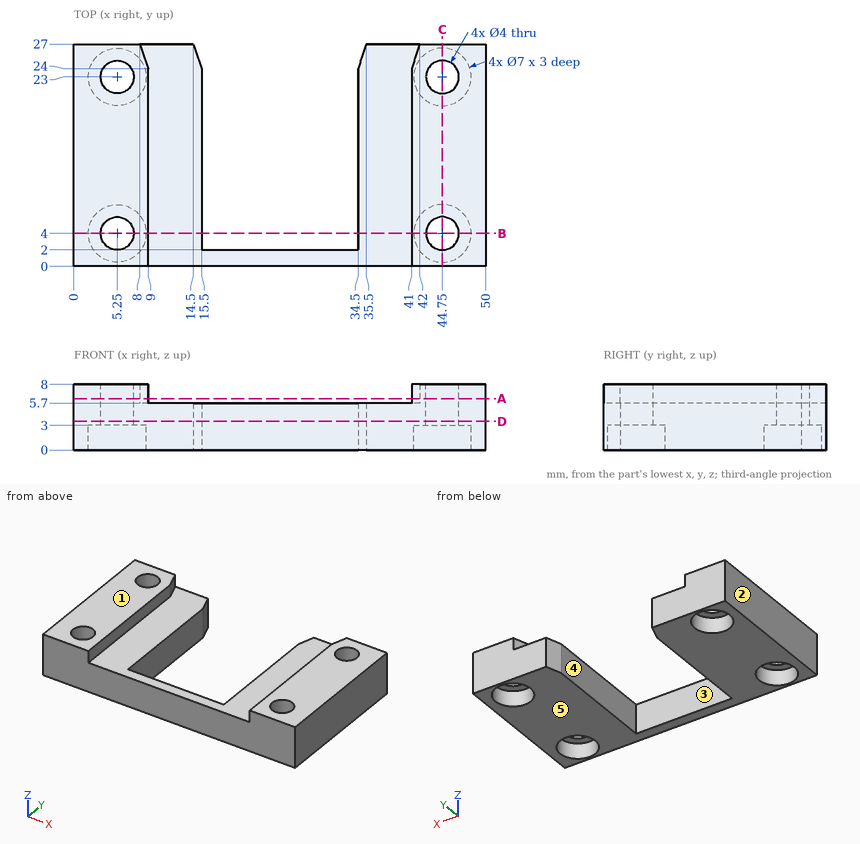
Job drawing, mm, ordinate dimensions from the low corner. One solid piece. A direction names the side the tool comes from. Round coordinates to 2 decimals unless told otherwise and drop trailing zeros. Loops run counter-clockwise (first coordinate to the right, second up) from the corner with the lowest first, then second, coordinate; pieces in that order, holes last.
(1) Cut at B-B (y = 4). Give the cut face in (x, z), plus the area to 3 significant figures.
(2) Cut at D-D (z = 3.5). Give the cut face in (x, y), plus the area to 3 significant figures.
(3) Drop flat-ended pins along their axis: pin 1 (4.5 mm diameter, centred on x = 26, z = 3.5, fed in from +Y); pin 2 (1.5 mm diameter, centred on x = 32, y = 20, fed in from -Z); pin 3 (3.5 mm diameter, centred on x = 6.5, y = 5, fed in from -Z). Give the stop position or say it passes through.
(4) Cut at A-A (z = 6.25). Give the cut face in (x, y).
(5) Two-plate mould, pull along X, no slides. Class the marked faces 1, 2 and 3: +X half, -X half, draft (parallel to the pull), parting line (faces both ways), or undercut.
(6) Wall check: line 1 along Y through (x, z) = (44.75, 2.2); line 2 along X through (y, z) = (4, 6.3); line 3 along Y through (x, z) = (44.75, 5.85). Give the ranges that are in metal, low to high.
(7) Cut at C-C (x = 44.75). Give the cut face in (y, z).
(8) Which spindle directions (+Z, -Z, +X, -X, +Y, -Y) get a long thin tool onto all of the face, cutting with end or side? Do the marked faces 4 and 5. Say none if no direction does.
Findings below:
1. outline: (0, 0) - (1.75, 0) - (1.75, 3) - (3.25, 3) - (3.25, 8) - (0, 8) - close; (7.25, 3) - (8.75, 3) - (8.75, 0) - (15.5, 0) - (15.5, 5.7) - (9, 5.7) - (9, 8) - (7.25, 8) - close; (34.5, 0) - (41.25, 0) - (41.25, 3) - (42.75, 3) - (42.75, 8) - (41, 8) - (41, 5.7) - (34.5, 5.7) - close; (46.75, 3) - (48.25, 3) - (48.25, 0) - (50, 0) - (50, 8) - (46.75, 8) - close
1. area: 136 mm2
2. outline: (0, 0) - (50, 0) - (50, 27) - (35.5, 27) - (34.5, 24) - (34.5, 2) - (15.5, 2) - (15.5, 24) - (14.5, 27) - (0, 27) - close; hole circle Ø4 at (5.25, 4); hole circle Ø4 at (5.25, 23); hole circle Ø4 at (44.75, 4); hole circle Ø4 at (44.75, 23)
2. area: 822 mm2
3. pin 1: stops at y = 2
3. pin 2: passes through
3. pin 3: stops at z = 3
4. outline: (0, 0) - (9, 0) - (9, 24) - (8, 27) - (0, 27) - close; (41, 0) - (50, 0) - (50, 27) - (42, 27) - (41, 24) - close; hole circle Ø4 at (5.25, 4); hole circle Ø4 at (5.25, 23); hole circle Ø4 at (44.75, 4); hole circle Ø4 at (44.75, 23)
5. face 1: draft
5. face 2: -X half
5. face 3: undercut
6. line 1: y = 0 to 0.5, 7.5 to 19.5, 26.5 to 27
6. line 2: x = 0 to 3.25, 7.25 to 9, 41 to 42.75, 46.75 to 50
6. line 3: y = 0 to 2, 6 to 21, 25 to 27
7. outline: (0, 0) - (0.5, 0) - (0.5, 3) - (2, 3) - (2, 8) - (0, 8) - close; (6, 3) - (7.5, 3) - (7.5, 0) - (19.5, 0) - (19.5, 3) - (21, 3) - (21, 8) - (6, 8) - close; (25, 3) - (26.5, 3) - (26.5, 0) - (27, 0) - (27, 8) - (25, 8) - close
8. face 4: +Z, -Z, +Y
8. face 5: -Z, +X, -X, +Y, -Y
